```python
from build123d import *

# Parameters (mm, degrees)
F0_R     = 32.5233232703
F1_DEPTH = 12.7
F2_R     = 19.4795835543
F3_DEPTH = 9.525
F4_SIZE2 = 7.62
F4_SIZE  = 6.35
F5_R     = 20.082572942
F6_DEPTH = 0.635
F8_DEPTH = 21.591
F9_DEPTH = 19.304


with BuildPart() as f1:
    # F0 (on Top) → F1 (new body)
    with BuildSketch(Plane.XY):
        with Locations((-16.1171220243, 12.0878415182)):
            Circle(F0_R)
    extrude(amount=F1_DEPTH)

    # F2 (on face) → F3 (join)
    with BuildSketch(Plane(origin=(0, 0, 0), x_dir=(1, 0, 0), z_dir=(0, 0, -1))):
        with Locations((-16.1171220243, -12.0878415182)):
            Circle(F2_R)
    extrude(amount=F3_DEPTH)

    # F4
    f4_edges = [f1.edges().sort_by_distance(p)[0] for p in [
        (-35.596706, 12.087842, -9.525),
    ]]
    f4_side = f1.faces().sort_by_distance((-16.117122, 12.087842, -9.525))[0]
    chamfer(f4_edges, length=F4_SIZE, length2=F4_SIZE2, reference=f4_side)

    # F5 (on face) → F6 (cut)
    with BuildSketch(Plane.XY.offset(12.7)):
        with Locations((-16.1171220243, 12.0878415182)):
            Circle(F5_R)
    extrude(amount=-F6_DEPTH, mode=Mode.SUBTRACT)

    # F7 (on face) → F8 (cut, through all)
    with BuildSketch(Plane.XY.offset(12.065)):
        with BuildLine():
            ThreePointArc((-39.3746949662, 12.0878415182), (-36.1996949662, 8.9128415182), (-33.0246949662, 12.0878415182))
            Line((-33.0246949662, 12.0878415182), (-39.3746949662, 12.0878415182))
        make_face()
        with BuildLine():
            Line((-39.3746949662, 12.0878415182), (-33.0246949662, 12.0878415182))
            ThreePointArc((-33.0246949662, 12.0878415182), (-36.1996949662, 15.2628415182), (-39.3746949662, 12.0878415182))
        make_face()
        with BuildLine():
            ThreePointArc((7.1404509177, 12.0878415182), (3.9654509177, 15.2628415182), (0.7904509177, 12.0878415182))
            Line((0.7904509177, 12.0878415182), (7.1404509177, 12.0878415182))
        make_face()
        with BuildLine():
            Line((7.1404509177, 12.0878415182), (0.7904509177, 12.0878415182))
            ThreePointArc((0.7904509177, 12.0878415182), (3.9654509177, 8.9128415182), (7.1404509177, 12.0878415182))
        make_face()
    extrude(amount=-F8_DEPTH, mode=Mode.SUBTRACT)

    # F7 (on face) → F9 (cut)
    with BuildSketch(Plane.XY.offset(12.065)):
        with BuildLine():
            ThreePointArc((-39.3746949662, 12.0878415182), (-36.1996949662, 8.9128415182), (-33.0246949662, 12.0878415182))
            Line((-33.0246949662, 12.0878415182), (-39.3746949662, 12.0878415182))
        make_face()
        with BuildLine():
            Line((-39.3746949662, 12.0878415182), (-33.0246949662, 12.0878415182))
            ThreePointArc((-33.0246949662, 12.0878415182), (-36.1996949662, 15.2628415182), (-39.3746949662, 12.0878415182))
        make_face()
        with BuildLine():
            ThreePointArc((7.1404509177, 12.0878415182), (3.9654509177, 15.2628415182), (0.7904509177, 12.0878415182))
            Line((0.7904509177, 12.0878415182), (7.1404509177, 12.0878415182))
        make_face()
        with BuildLine():
            Line((7.1404509177, 12.0878415182), (0.7904509177, 12.0878415182))
            ThreePointArc((0.7904509177, 12.0878415182), (3.9654509177, 8.9128415182), (7.1404509177, 12.0878415182))
        make_face()
    extrude(amount=F9_DEPTH, mode=Mode.SUBTRACT)


solid = f1.part
```
Could you check a few things on this model? Use its own coordinates, in mm. A direction names the side the tool comes from. Round coordinates to 2 decimals unless told otherwise and drop trailing zeros. Write each loop counter-clockwise with the first axis right and the second up, starting at its lowest first coordinate (ties: lowest second). Pieces come first, ordered by that corner, then holes. Notation, with made-up numbers: M -4,-19 L 2,-19 A29 ccw 2,15 Z; hole C 31.5,85 d2. An arc over 180 degrees is marked long. Write each question's results on one line, items separated by ' | '. Start each with the question number.
1. Imagine slicing it at C-C on y = -13.5. List the corners of the cut face in (x, z) for me.
2. I need wall thicknesses on L1, parallel to Z at x = -1, y = 25.5; L2, parallel to Z at x = -10, y = 15.5 (3 decimals); L3, parallel to Y at x = -37, z = 6. Which ranges of each line are inside material? Lowest first, please. Write a range as from..to.
3. Imagine slicing it at B-B on z = -8. List the corners of the cut face in (x, y) for me, and give its area (3 significant figures).
4. Imagine slicing it at D-D on z = 4.25. List the corners of the cut face in (x, y) for me (3 decimals).
5. I'm going to push flat-ended pins straight in: pin 1 Ø10 at (x, y) = (-36.2, 12.09) entering from +Z; pin 2 Ø3 at (x, z) = (-10, 8) entering from -Y; pin 3 Ø6 at (x, z) = (-2.5, -1) entering from -Y; pin 4 Ø10 at (y, z) = (20.5, 8) entering from +X. Where does each tip first touch, or does it pass through?
6. Imagine slicing it at A-A on x = -38. List the corners of the cut face in (y, z) for me, and give its area (3 significant figures).
7. On a 3-axis mill with a long thin cutter (end or side, diameter ignored), from which of +Z, -Z, +X, -X, +Y, -Y can I reach the whole of each face in a straight line? I mean faces 1 (the face through (-2, -2, 0)), 2 (the face through (-16.51, -7.99, 12.39)), 3 (the face through (-16.502, 31.564, -0.939)), 4 (the face through (-33.17, 13.04, 5.94)). Say none if no direction works.
8. Thinking about a two-plate mould opening in X: for faces 5 (the face through (-16, 12, -9.525)), 6 (the face through (-15.72, 32.166, 12.387)), 7 (the face through (-15.732, -7.388, -0.939)), which applies, +X half, -X half, draft (parallel to the pull), parting line (faces both ways), or undercut?
Result sheet:
1) outline: M -36.19,0 L 3.96,0 L 3.96,12.7 L -36.19,12.7 Z
2) L1: z = 0..12.7 | L2: z = -9.525..12.065 | L3: y = -12.85..9.02, 15.16..37.02
3) outline: C -16.12,12.09 d28.8 | area: 651 mm^2
4) outline: C -16.117,12.088 d65.047; hole C -36.2,12.088 d6.35; hole C 3.965,12.088 d6.35
5) pin 1: stops at z = 12.7 | pin 2: stops at y = -20.11 | pin 3: stops at y = -18.59 | pin 4: stops at x = 16.23
6) outline: M -11.97,0 L 9.47,0 L 9.47,12.7 L -11.97,12.7 Z; M 14.7,0 L 36.15,0 L 36.15,12.7 L 14.7,12.7 Z | area: 545 mm^2
7) face 1: -Z | face 2: +Z | face 3: -Z, +Y | face 4: +Z, -Z
8) face 5: draft | face 6: undercut | face 7: parting line
